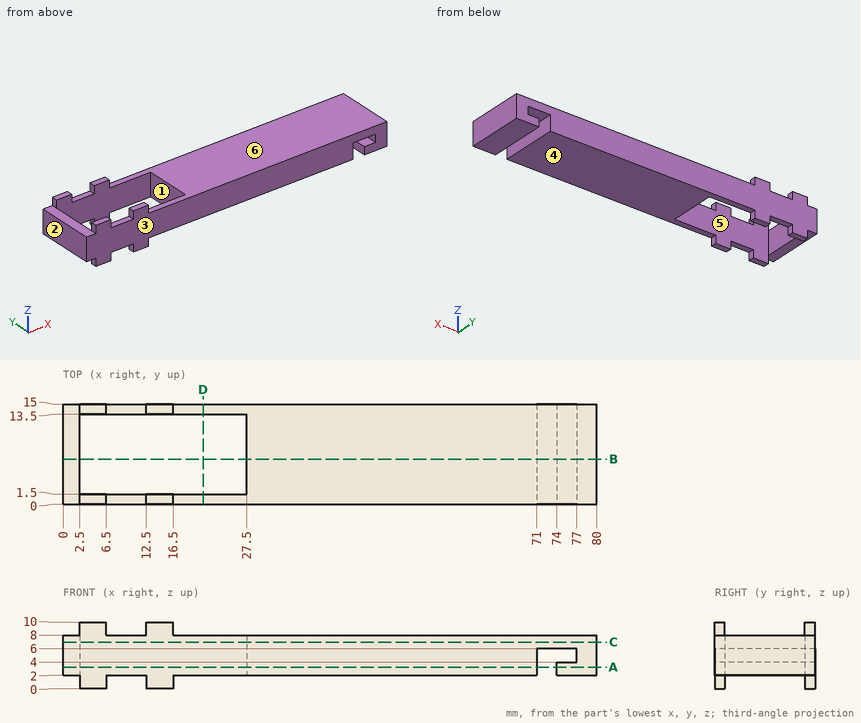
Check sheet for the drawn part. Datum: minimum x, y, z corner. Units: mm. A direction names the side the tool comes from. Round coordinates to 2 decimals unless told otherwise and drop trailing zeros. Order: outer loops, then holes, each group sorted by start corner. A loop starts at its lowest first (then second) coordinate and runs counter-clockwise, first axis right, second up. Notation, with made-up numbers: M 65.5,-10.5 L 111.5,-10.5 A32 ccw 111.5,18.5 Z; hole C 23.5,-35.75 d7. An arc over 180 degrees is marked long. Answer in a Markdown table with one row per item.
(1) Gauge pin test, flat ends, axial feed: pin 1 (4.5 mm diameter, centred on x = 63, y = 5.5, fed in from +Z); pin 2 (7.5 mm diameter, centred on x = 44, y = 4, fed in from -Z); pin 3 (1.2 mm diameter, centred on y = 14, z = 9, fed in from -X); pin 4 (2 mm diameter, centred on x = 63.5, z = 1.5, fed in from +Y). Record the tip position at first contact, or that the pin passes through.
Findings:
| item | result |
|---|---|
| pin 1 | stops at z = 8 |
| pin 2 | stops at z = 2 |
| pin 3 | stops at x = 2.5 |
| pin 4 | stops at y = 15 |
(2) Section check D-D on x = 21. Record the boundary of the cut face in (y, z), plus the area to 3 significant figures.
Findings:
| item | result |
|---|---|
| outline | M 0,2 L 1.5,2 L 1.5,8 L 0,8 Z; M 13.5,2 L 15,2 L 15,8 L 13.5,8 Z |
| area | 18.0 mm^2 |
(3) Section check B-B on y = 6.75. Record the boundary of the cut face in (x, z).
Findings:
| item | result |
|---|---|
| outline | M 0,2 L 2.5,2 L 2.5,8 L 0,8 Z; M 27.5,2 L 71,2 L 71,6 L 77,6 L 77,4 L 74,4 L 74,2 L 80,2 L 80,8 L 27.5,8 Z |
(4) Section check C-C on z = 7. Record the boundary of the cut face in (x, y), plus the area to 3 significant figures.
Findings:
| item | result |
|---|---|
| outline | M 0,0 L 80,0 L 80,15 L 0,15 Z; hole M 2.5,1.5 L 27.5,1.5 L 27.5,13.5 L 2.5,13.5 Z |
| area | 900 mm^2 |
(5) Draft check along X on the marked faces 1, 2 and 3. Enter one of: +X half, -X half, draft (parallel to the pull), parting line (faces both ways), or undercut.
Findings:
| item | result |
|---|---|
| face 1 | undercut |
| face 2 | -X half |
| face 3 | draft |
(6) Set-up check for the marked faces 4, 5 and 6: record each of +Z, -Z, +X, -X, +Y, -Y from which the full face is reachable in a straight line by a thin tool's end or side.
Findings:
| item | result |
|---|---|
| face 4 | -Z, +X, +Y, -Y |
| face 5 | +Z, -Z |
| face 6 | +Z, +X, +Y, -Y |
(7) Section check A-A on z = 3.25. Record the boundary of the cut face in (x, y).
Findings:
| item | result |
|---|---|
| outline | M 0,0 L 71,0 L 71,15 L 0,15 Z; M 74,0 L 80,0 L 80,15 L 74,15 Z; hole M 2.5,1.5 L 27.5,1.5 L 27.5,13.5 L 2.5,13.5 Z |
(8) Material ranges on line 1 along X through (y, z) = (5.5, 2.5); line 2 along X through (y, z) = (2, 5.25); line 3 along Y through (x, z) = (14, 2.25), recorded low to high. Write a range as from..to.
Findings:
| item | result |
|---|---|
| line 1 | x = 0..2.5, 27.5..71, 74..80 |
| line 2 | x = 0..2.5, 27.5..71, 77..80 |
| line 3 | y = 0..1.5, 13.5..15 |
